Work out the finished part from the listing and answer in its coordinate system (mm). Face numbers are marked on the shaded views. A direction names the side the tool comes from. Give positions to 0.01 mm unless a question says otherwise; leave off trailing zeros. Order: outer loops, then holes, each group sorted by start corner. A loop starts at its lowest first (then second) coordinate and runs counter-clockwise, first axis right, second up. Notation, with made-up numbers: M 9.5,-15.5 L 48.5,-15.5 A18 cw 48.5,9.5 Z; hole C -10.5,24.25 d4. An arc over 180 degrees is marked long. One line per item, written item: value.
from build123d import *

# Parameters (mm, degrees)
SKETCH1_R           = 17.5
MOTOR_BASE_DEPTH    = 60
SKETCH2_R           = 2.5
SHAFT_DEPTH         = 20
SKETCH3_R           = 6.5
BOSS_EXTRUDE3_DEPTH = 2
SKETCH4_R           = 1
CUT_EXTRUDE1_DEPTH  = 2.54


with BuildPart() as part:
    # Sketch1 → Motor-Base (new body)
    with BuildSketch(Plane.XY):
        Circle(SKETCH1_R)
    extrude(amount=MOTOR_BASE_DEPTH)

    # Sketch2 → Shaft (add)
    with BuildSketch(Plane.XY.offset(60)):
        with Locations((0, -5.5)):
            Circle(SKETCH2_R)
    extrude(amount=SHAFT_DEPTH)

    # Sketch3 → Boss-Extrude3 (add)
    with BuildSketch(Plane.XY.offset(60)):
        with Locations((0, -5.5)):
            Circle(SKETCH3_R)
    extrude(amount=BOSS_EXTRUDE3_DEPTH)

    # Sketch4 → Cut-Extrude1 (cut)
    with BuildSketch(Plane.XY.offset(60)):
        with Locations((9.759593791, -5.5)):
            Circle(SKETCH4_R)
    extrude(amount=-CUT_EXTRUDE1_DEPTH, mode=Mode.SUBTRACT)


solid = part.part
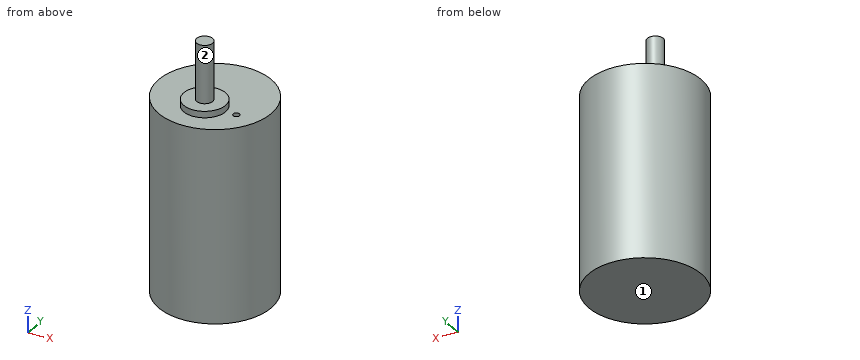
(1) Which of the six approach directions +Z, -Z, +X, -X, +Y, -Y give full straight-line access (tool end or side, diameter ignored) to the marked faces 1 and 2?
Findings:
face 1: -Z, +X, -X, +Y, -Y
face 2: +Z
(2) Section A-A, the plane x = 0 is taken. Give the vertices of the cut face in (y, z).
Findings:
outline: M -17.5,0 L 17.5,0 L 17.5,60 L 1,60 L 1,62 L -3,62 L -3,80 L -8,80 L -8,62 L -12,62 L -12,60 L -17.5,60 Z
(3) Find the intervals of material crossed by probe 1 along Z at (x, y) = (3, -3); probe 2 along Z at (x, y) = (12, 8.5); probe 3 along X at (y, z) = (-5, 58), in increasing order. Write a range as from..to.
Findings:
probe 1: z = 0..62
probe 2: z = 0..60
probe 3: x = -16.77..8.89, 10.63..16.77
(4) Section B-B, the plane y = -5.5 is taken. Give the vertices of the cut face in (x, z), then the cut area to 3 significant figures.
Findings:
outline: M -16.61,0 L 16.61,0 L 16.61,60 L 10.76,60 L 10.76,57.46 L 8.76,57.46 L 8.76,60 L 6.5,60 L 6.5,62 L 2.5,62 L 2.5,80 L -2.5,80 L -2.5,62 L -6.5,62 L -6.5,60 L -16.61,60 Z
area: 2,100 mm^2
(5) Section D-D, the plane y = 0 is taken. Give the vertices of the cut face in (x, z).
Findings:
outline: M -17.5,0 L 17.5,0 L 17.5,60 L 3.46,60 L 3.46,62 L -3.46,62 L -3.46,60 L -17.5,60 Z
(6) Given P1, Ø1.6, axis at x = 9.5, y = -6, coming from the +Z side; P2, Ø12, axis at y = 3.5, z = 42.5, coming from the +X side; P3, Ø1.5, axis at y = -11, z = 52.5, coming from the -X side; P4, Ø3, axis at y = -12.5, z = 19, coming from the -X side, each flat-ended and moving along its own axis, determine where each tip first touches the part or whether it passes through.
Findings:
P1: stops at z = 60
P2: stops at x = 17.5
P3: stops at x = -14.18
P4: stops at x = -13.61
(7) Section C-C, the plane z = 69.5 is taken. Give the vertices of the cut face in (x, y).
Findings:
outline: C 0,-5.5 d5
